Work out the finished part from the listing and answer in its coordinate system (mm). A direction names the side the tool comes from. Round coordinates to 2 decimals unless told otherwise and drop trailing zeros. Write each loop counter-clockwise with the first axis right and the second up, starting at its lowest first coordinate (ties: lowest second). Pieces come first, ordered by that corner, then holes. Notation, with made-up numbers: M -31,15.25 L -2,15.25 A20 cw -2,38.25 Z; hole C 3,39 d8. An arc over 180 degrees is marked long. One line per item, written item: value. Start each with the question number.
Q1. Consider probe 1 along Y at (x, z) = (-27, 1.4); probe 2 along Y at (x, z) = (15.5, 1.85); probe 3 along Y at (x, z) = (17, 2.25). Determine where each line is inside the solid, lowest interval first.
Q2. Given pin 1 Ø1.5 at (x, z) = (-26.5, 3) entering from +Y; pin 2 Ø2 at (x, y) = (-17.01, -6) entering from -Z; pin 3 Ø0.9 at (x, z) = (11, 2.5) entering from -Y; pin 4 Ø2.5 at (x, z) = (-26.5, 2.5) entering from -Y, each flat-ended and moving along its own axis, determine where each tip first touches the part or whether it passes through.
Q3. Find section B-B (z = 1.85). Write down the section's boundary in (x, y).
Q4. A tool of negligible diameter and unlimited length cuts with its end or side. For faces 4 (the flat face through (11, -5, 2)), 5 (the flat face through (17.589, -7.144, 2.465)), 6 (the flat face through (-26, -9.527, 2)), from which of +Z, -Z, +X, -X, +Y, -Y can it reach the whole face along a straight path? Write none if from no direction.
Q5. Find section A-A (x = -27). Write down the section's boundary in (y, z), and give its area (3 significant figures).
Q6. The mould has two halves that part along Y. Classify faces 1 (the cylindrical face through (-25.95, -9.24, 0.3)), 2 (the cylindrical face through (23.09, -4.03, 2.46)), 3 (the cylindrical face through (-9.87, -2.03, 4.7)): released by +Y, released by -Y, zero draft, split by the parting line, or undercut.
from build123d import *

# Parameters (mm, degrees)
BOSS_EXTRUDE1_DEPTH = 5
FILLET1_R           = 1
SKETCH2_R           = 1.75
CUT_EXTRUDE1_DEPTH  = 35.054632191


with BuildPart() as part:
    # Sketch1 → Boss-Extrude1 (new body)
    with BuildSketch(Plane.XY):
        with BuildLine():
            Line((4.374433176, 0), (26.535898385, 0))
            ThreePointArc((26.535898385, 0), (28.267949192, -1), (28.267949192, -3))
            Line((28.267949192, -3), (21.732050808, -14.320508076))
            ThreePointArc((21.732050808, -14.320508076), (20, -15.320508076), (18.267949192, -14.320508076))
            Line((18.267949192, -14.320508076), (13.464101615, -6))
            ThreePointArc((13.464101615, -6), (12.732050808, -5.267949192), (11.732050808, -5))
            Line((11.732050808, -5), (10.570646977, -5))
            ThreePointArc((10.570646977, -5), (6.21285984, -5.190265095), (1.888238094, -5.759612349))
            Line((1.888238094, -5.759612349), (-15.167092312, -8.766927265))
            ThreePointArc((-15.167092312, -8.766927265), (-19.491714058, -9.336274519), (-23.849501195, -9.526539614))
            Line((-23.849501195, -9.526539614), (-28, -9.526539614))
            ThreePointArc((-28, -9.526539614), (-29.414213562, -8.940753177), (-30, -7.526539614))
            Line((-30, -7.526539614), (-30, -5.526539614))
            ThreePointArc((-30, -5.526539614), (-29.414213562, -4.112326052), (-28, -3.526539614))
            Line((-28, -3.526539614), (-24.374433176, -3.526539614))
            ThreePointArc((-24.374433176, -3.526539614), (-20.016646039, -3.336274519), (-15.692024293, -2.766927265))
            Line((-15.692024293, -2.766927265), (-4.307975707, -0.759612349))
            ThreePointArc((-4.307975707, -0.759612349), (0.016646039, -0.190265095), (4.374433176, 0))
        make_face()
        with BuildLine():
            Line((21.732050808, -8.320508076), (23.07179677, -6))
            ThreePointArc((23.07179677, -6), (23.07179677, -4), (21.339745962, -3))
            Line((21.339745962, -3), (18.660254038, -3))
            ThreePointArc((18.660254038, -3), (16.92820323, -4), (16.92820323, -6))
            Line((16.92820323, -6), (18.267949192, -8.320508076))
            ThreePointArc((18.267949192, -8.320508076), (20, -9.320508076), (21.732050808, -8.320508076))
        make_face(mode=Mode.SUBTRACT)
    extrude(amount=BOSS_EXTRUDE1_DEPTH)

    # Fillet1
    fillet1_edges = [part.edges().sort_by_distance(p)[0] for p in [
        (-19.491714058, -9.336274519, 5),
        (-6.639427109, -7.263269807, 5),
        (-30, -6.526539614, 0),
        (-29.414213562, -4.112326052, 0),
        (-26.187216588, -3.526539614, 0),
        (-20.016646039, -3.336274519, 0),
        (-10, -1.763269807, 0),
        (0.016646039, -0.190265095, 0),
        (15.455165781, 0, 0),
        (28.267949192, -1, 0),
        (25, -8.660254038, 0),
        (6.21285984, -5.190265095, 5),
        (20, -15.320508076, 0),
        (15.866025404, -10.160254038, 0),
        (12.732050808, -5.267949192, 0),
        (11.151348892, -5, 0),
        (6.21285984, -5.190265095, 0),
        (-6.639427109, -7.263269807, 0),
        (-19.491714058, -9.336274519, 0),
        (-25.924750598, -9.526539614, 0),
        (-29.414213562, -8.940753177, 0),
        (11.151348892, -5, 5),
        (12.732050808, -5.267949192, 5),
        (15.866025404, -10.160254038, 5),
        (20, -15.320508076, 5),
        (25, -8.660254038, 5),
        (28.267949192, -1, 5),
        (15.455165781, 0, 5),
        (-29.414213562, -8.940753177, 5),
        (0.016646039, -0.190265095, 5),
        (-10, -1.763269807, 5),
        (-20.016646039, -3.336274519, 5),
        (-26.187216588, -3.526539614, 5),
        (-29.414213562, -4.112326052, 5),
        (-30, -6.526539614, 5),
        (-25.924750598, -9.526539614, 5),
    ]]
    fillet(fillet1_edges, radius=FILLET1_R)

    # Sketch2 → Cut-Extrude1 (cut, through all)
    with BuildSketch(Plane.XY.offset(5)):
        with Locations((-17.013893068, -5.999597174)):
            Circle(SKETCH2_R)
        with Locations((-27, -6.526539614)):
            Circle(SKETCH2_R)
    extrude(amount=-CUT_EXTRUDE1_DEPTH, mode=Mode.SUBTRACT)


solid = part.part
The answers:
1. probe 1: -9.53 to -8.28, -4.78 to -3.53
1. probe 2: -9.53 to 0
1. probe 3: -12.12 to -6.12, -3.88 to 0
2. pin 1: y = -3.53
2. pin 2: through
2. pin 3: y = -5
2. pin 4: y = -9.53
3. outline: M -30,-7.53 A2 ccw -28,-9.53 L -23.85,-9.53 A50 ccw -15.17,-8.77 L 1.89,-5.76 A50 cw 10.57,-5 L 11.73,-5 A2 cw 13.46,-6 L 18.27,-14.32 A2 ccw 21.73,-14.32 L 28.27,-3 A2 ccw 26.54,0 L 4.37,0 A50 ccw -4.31,-0.76 L -15.69,-2.77 A50 cw -24.37,-3.53 L -28,-3.53 A2 ccw -30,-5.53 Z; hole C -27,-6.53 d3.5; hole C -17.01,-6 d3.5; hole M 16.93,-6 L 18.27,-8.32 A2 ccw 21.73,-8.32 L 23.07,-6 A2 ccw 21.34,-3 L 18.66,-3 A2 ccw Z
4. face 4: +Z, -Z, -Y
4. face 5: +Z, -Z
4. face 6: +Z, -Z, -X, -Y
5. outline: M -9.53,1 A1 ccw -8.53,0 L -8.28,0 L -8.28,5 L -8.53,5 A1 ccw -9.53,4 Z; M -4.78,0 L -4.53,0 A1 ccw -3.53,1 L -3.53,4 A1 ccw -4.53,5 L -4.78,5 Z
5. area: 11.6 mm2
6. face 1: released by -Y
6. face 2: undercut
6. face 3: released by +Y
